Autodesk Fusion 360 part; units mm, degrees
sketch "Base Sketch" plane through (0, 0, 0) normal (0, 0, 1) x (1, 0, 0)
  line L0 (57, 32) -> (-57, 32)
  line L1 (-57, -32) -> (57, -32)
  circle A0 centre (57, 0) radius 11
  circle A1 centre (-57, 0) radius 11.0308
  arc A2 (-55.5967, 32) -> (-55.5967, -32) centre (-57, 0) ccw
  arc A3 (57, -32) -> (57, 32) centre (57, 0) ccw
  dimension "d1" = 114
  dimension "d2" = 64
  dimension "d3" = 64.0615
extrude "Extrude1" add sketch "Base Sketch" along normal blind 19
sketch "Cube Sketch" plane through (0, 0, 19) normal (0, 0, 1) x (-1, 0, 0)
  circle A0 centre (57, 0) radius 11.0308
  circle A1 centre (-57, 0) radius 11
  arc A2 (-57, 32) -> (-57, -32) centre (-57, 0) ccw
  line L0 (-57, -32) -> (55.5967, -32)
  arc A3 (55.5967, -32) -> (55.5967, 32) centre (57, 0) ccw
  line L1 (55.5967, 32) -> (-57, 32)
  line L2 (32, 32) -> (-32, 32)
  line L3 (-32, 32) -> (-32, -32)
  line L4 (-32, -32) -> (32, -32)
  line L5 (32, -32) -> (32, 32)
  line L6 (32, 32) -> (-32, -32) construction
  line L7 (-32, 32) -> (32, -32) construction
  line L8 (18.7079, 32) -> (-19.2921, 32)
  line L9 (-19.2921, 32) -> (-19.2921, -19)
  line L10 (-19.2921, -19) -> (18.7079, -19)
  line L11 (18.7079, -19) -> (18.7079, 32)
  dimension "d8" = 64
  dimension "d9" = 64
  dimension "d10" = 38
  dimension "d11" = 51
sketch "Triangle Sketch" plane through (0, 0, 0) normal (1, 0, 0) x (0, 1, 0)
  line L0 (-32, 19) -> (19, 19)
  line L1 (19, 19) -> (19, 64)
  line L2 (19, 64) -> (-32, 19)
  dimension "d12" = 51
  dimension "d13" = 45
extrude "Extrude2" add sketch "Triangle Sketch" along normal mid plane 38
extrude "Extrude3" add sketch "Cube Sketch" along normal blind 45 contours L0 L1 L2 L3 L4 L5 L9 L10 L11
equation "d2 = ( 32 * 2 ) * 1 mm"
equation "d13 = 64 mm - 19 mm"
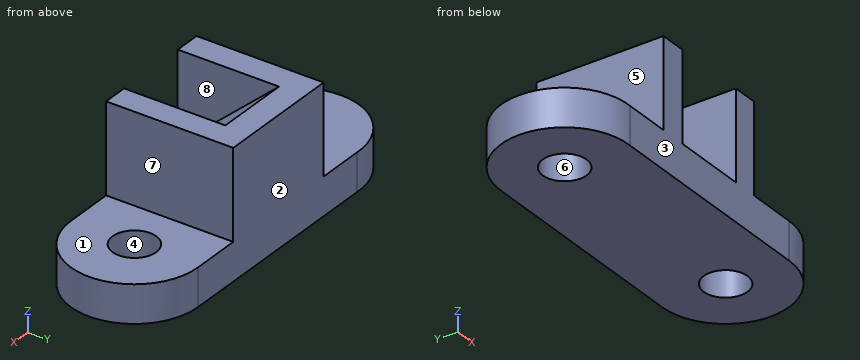
Read the model definition and answer for the solid it produces. Units are mm, in the model's axes. Face numbers are marked on the shaded views. A direction names the side the tool comes from. Coordinates: 2 decimals unless noted, no trailing zeros. Order: outer loops, then holes, each group sorted by start corner. A loop starts at its lowest first (then second) coordinate and runs counter-clockwise, first axis right, second up. Notation, with made-up numbers: M -37.5,-18 L -33.5,-18 A14 ccw -33.5,-13 Z; hole C 20,15 d2. An arc over 180 degrees is marked long. Put each result on its own line as item: value. Start each with the question number.
Item 1: Section B-B, the plane z = 7.5 is taken. Determine the outline of the cut face in (x, y).
Item 2: Section C-C, the plane z = 46 is taken. Determine the outline of the cut face in (x, y).
Item 3: Consider probe 1 along X at (y, z) = (-15.5, 60); probe 2 along Y at (x, z) = (-57, 8); probe 3 along X at (y, z) = (-8, 26.5). Determine where each line is inside the solid, lowest interval first. Write a range as [from, to].
Item 4: Section A-A, the plane y = -5 is taken. Determine the outline of the cut face in (x, z).
Item 5: Given pin 1 Ø1.5 at (y, z) = (-5.5, 57.5) entering from -X; pin 2 Ø3 at (y, z) = (12, 10) entering from +X; pin 3 Ø1.5 at (y, z) = (-2, 42.5) entering from +X, each flat-ended and moving along its own axis, determine where each tip first touches the part or whether it passes through.
Item 6: The mould has two halves that part along Y. Classify the marked faces 1, 2, 3 and 4: +Y half, -Y half, draft (parallel to the pull), parting line (faces both ways), or undercut.
Item 7: For the marked faces 5, 6, 7 and 8, determine the directions among +Z, -Z, +X, -X, +Y, -Y from which every point of the face is accessible in a straight line to the end or side of a thin tool.
Computed:
1. outline: M -55.6,-32 L 57,-32 A32 ccw 57,32 L -55.6,32 A32.03 ccw long Z; hole C -57,0 d22.06; hole C 57,0 d22
2. outline: M -32,-32 L -18.71,-32 L -18.71,-1.4 L 19,-1.4 L 19,19 L 19.29,19 L 19.29,-32 L 32,-32 L 32,32 L -32,32 Z
3. probe 1: x = [-32, -18.71], [19.29, 32]
3. probe 2: y = [-32.03, -11.03], [11.03, 32.03]
3. probe 3: x = [-32, 19], [19.29, 32]
4. outline: M -88.64,0 L -66.83,0 L -66.83,19 L -88.64,19 Z; M -47.17,0 L 47.2,0 L 47.2,19 L 32,19 L 32,64 L 19.29,64 L 19.29,19 L 19,19 L 19,42.82 L -18.71,42.82 L -18.71,64 L -32,64 L -32,19 L -47.17,19 Z; M 66.8,0 L 88.61,0 L 88.61,19 L 66.8,19 Z
5. pin 1: stops at x = -32
5. pin 2: stops at x = 87.23
5. pin 3: stops at x = 32
6. face 1: draft
6. face 2: +Y half
6. face 3: -Y half
6. face 4: undercut
7. face 5: +Z, -X, +Y, -Y
7. face 6: +Z, -Z
7. face 7: +Z, +X, +Y, -Y
7. face 8: +Z, -Y
